Autodesk Fusion 360 part; units mm, degrees
sketch "Sketch1" plane through (0, 0, 0) normal (0, 0, 1) x (1, 0, 0)
  line L0 (0, 0) -> (35, 0)
  line L1 (35, 0) -> (35, 35)
  line L2 (35, 35) -> (0, 35)
  line L3 (0, 35) -> (0, 0)
  dimension "d1" = 35
  dimension "d2" = 35
extrude "Extrude1" add sketch "Sketch1" along normal blind 3
sketch "Sketch2" plane through (0, 0, 3) normal (0, 0, 1) x (-1, 0, 0)
  line L0 (0, -35) -> (0, 0)
  line L1 (0, 0) -> (-35, 0)
  line L2 (-35, 0) -> (-35, -35)
  line L3 (-35, -35) -> (0, -35)
  line L4 (-10, -35) -> (-35, -35)
  line L5 (-35, -35) -> (-35, -17.5)
  line L6 (-35, -17.5) -> (-10, -17.5)
  line L7 (-10, -17.5) -> (-10, -35)
  dimension "d5" = 25
  dimension "d6" = 17.5
extrude "Extrude2" cut sketch "Sketch2" against normal blind 3 contours L2 L3 L4 L5 L6 L7
sketch "Sketch6" plane through (0, 0, 3) normal (0, 0, 1) x (-1, 0, 0)
  line L0 (-35, -17.5) -> (-10, -17.5)
  line L1 (-10, -17.5) -> (-10, -35)
  line L2 (-10, -35) -> (0, -35)
  line L3 (0, -35) -> (0, 0)
  line L4 (0, 0) -> (-35, 0)
  line L5 (-35, 0) -> (-35, -17.5)
  line L6 (-10, -17.5) -> (-14, -17.5)
  line L7 (-14, -17.5) -> (-14, 0)
  line L8 (-14, 0) -> (-10, 0)
  line L9 (-10, 0) -> (-10, -17.5)
  dimension "d23" = 4
  dimension "d24" = 17.5
extrude "Extrude6" add sketch "Sketch6" along normal blind 6 contours L0 L4 L6 L7 L8 L9
extrude "Extrude7" cut 1 faces at (35, 5.8333, 1) along direction (-1, 0, 0) blind 5
sketch "Sketch7" plane through (0, 0, 3) normal (0, 0, 1) x (-1, 0, 0)
  line L0 (-30, 0) -> (-30, -17.5)
  line L1 (-30, -17.5) -> (-14, -17.5)
  line L2 (-14, -17.5) -> (-14, 0)
  line L3 (-14, 0) -> (-30, 0)
  line L4 (-30, -17.5) -> (-26, -17.5)
  line L5 (-26, -17.5) -> (-26, 0)
  line L6 (-26, 0) -> (-30, 0)
  line L7 (-30, 0) -> (-30, -17.5)
  dimension "d29" = 4
  dimension "d30" = 17.5
extrude "Extrude8" add sketch "Sketch7" along normal blind 6 contours L0 L1 L3 L4 L5 L6 L7
extrude "Extrude9" add 1 faces at (28.6667, 17.5, 4) along direction (0, 1, 0) blind 3.5
sketch "Sketch8" plane through (14, 0, 0) normal (1, 0, 0) x (0, 1, 0)
  line L0 (0, 3) -> (21, 3)
  line L1 (21, 3) -> (21, 9)
  line L2 (21, 9) -> (0, 9)
  line L3 (0, 9) -> (0, 3)
  line L4 (0, 7) -> (21, 7)
  line L5 (21, 7) -> (21, 5)
  line L6 (21, 5) -> (0, 5)
  line L7 (0, 5) -> (0, 7)
  dimension "d35" = 2
  dimension "d36" = 2
extrude "Extrude10" cut sketch "Sketch8" against normal blind 2 contours L1 L3 L4 L5 L6 L7
sketch "Sketch9" plane through (26, 0, 0) normal (-1, 0, 0) x (0, -1, 0)
  line L0 (-21, 3) -> (0, 3)
  line L1 (0, 3) -> (0, 9)
  line L2 (0, 9) -> (-21, 9)
  line L3 (-21, 9) -> (-21, 3)
  line L4 (-21, 7) -> (0, 7)
  line L5 (0, 7) -> (0, 5)
  line L6 (0, 5) -> (-21, 5)
  line L7 (-21, 5) -> (-21, 7)
  dimension "d39" = 2
  dimension "d40" = 2
extrude "Extrude11" cut sketch "Sketch9" against normal blind 2 contours L1 L3 L4 L5 L6 L7
sketch "Sketch10" plane through (0, 0, 5) normal (0, 0, 1) x (-1, 0, 0)
  line L0 (-26, -21) -> (-26, 0)
  line L1 (-26, 0) -> (-28, 0)
  line L2 (-28, 0) -> (-28, -21)
  line L3 (-28, -21) -> (-26, -21)
  line L4 (-26, 0) -> (-28, 0)
  line L5 (-28, 0) -> (-28, -2)
  line L6 (-28, -2) -> (-26, -2)
  line L7 (-26, -2) -> (-26, 0)
  dimension "d43" = 2
  dimension "d44" = 2
extrude "Extrude12" add sketch "Sketch10" along normal blind 2 contours L0 L1 L2 L4 L5 L6 L7
sketch "Sketch11" plane through (0, 0, 5) normal (0, 0, 1) x (-1, 0, 0)
  line L0 (-14, 0) -> (-14, -21)
  line L1 (-14, -21) -> (-12, -21)
  line L2 (-12, -21) -> (-12, 0)
  line L3 (-12, 0) -> (-14, 0)
  line L4 (-14, 0) -> (-12, 0)
  line L5 (-12, 0) -> (-12, -2)
  line L6 (-12, -2) -> (-14, -2)
  line L7 (-14, -2) -> (-14, 0)
  dimension "d47" = 2
  dimension "d48" = 2
extrude "Extrude13" add sketch "Sketch11" along normal blind 2 contours L0 L2 L3 L4 L5 L6 L7
sketch "Sketch14" plane through (0, 21, 0) normal (0, 1, 0) x (-1, 0, 0)
  line L0 (-26, 5) -> (-28, 5)
  line L1 (-28, 5) -> (-28, 7)
  line L2 (-28, 7) -> (-26, 7)
  line L3 (-26, 7) -> (-26, 9)
  line L4 (-26, 9) -> (-30, 9)
  line L5 (-30, 9) -> (-30, 0)
  line L6 (-30, 0) -> (-10, 0)
  line L7 (-10, 0) -> (-10, 3)
  line L8 (-10, 3) -> (-10, 9)
  line L9 (-10, 9) -> (-14, 9)
  line L10 (-14, 9) -> (-14, 7)
  line L11 (-14, 7) -> (-12, 7)
  line L12 (-12, 7) -> (-12, 5)
  line L13 (-12, 5) -> (-14, 5)
  line L14 (-14, 5) -> (-14, 3)
  line L15 (-14, 3) -> (-26, 3)
  line L16 (-26, 3) -> (-26, 5)
  line L17 (-10, 3) -> (-30, 3)
  line L18 (-30, 3) -> (-30, 0)
  line L19 (-30, 0) -> (-10, 0)
  line L20 (-10, 0) -> (-10, 3)
  dimension "d61" = 20
extrude "Extrude17" add sketch "Sketch14" along normal blind 10 contours L5 L6 L7 L15 L17 L18 L19 L20
extrude "Extrude18" cut 1 faces at (0, 23.3333, 1) along direction (1, 0, 0) blind 10
sketch "Sketch15" plane through (10, 0, 0) normal (-1, 0, 0) x (0, -1, 0)
  line L0 (0, 0) -> (0, 9)
  line L1 (0, 9) -> (-21, 9)
  line L2 (-21, 9) -> (-21, 3)
  line L3 (-21, 3) -> (-31, 3)
  line L4 (-31, 3) -> (-31, 0)
  line L5 (-31, 0) -> (0, 0)
  line L6 (-21, 3) -> (-31, 3)
  line L7 (-31, 3) -> (-31, 0)
  line L8 (-31, 0) -> (-21, 0)
  line L9 (-21, 0) -> (-21, 3)
extrude "Extrude19" add sketch "Sketch15" along normal blind 8 contours L3 L4 L5 L6 L7 L8 L9
sketch "Sketch16" plane through (30, 0, 0) normal (1, 0, 0) x (0, 1, 0)
  line L0 (21, 9) -> (0, 9)
  line L1 (0, 9) -> (0, 0)
  line L2 (0, 0) -> (31, 0)
  line L3 (31, 0) -> (31, 3)
  line L4 (31, 3) -> (21, 3)
  line L5 (21, 3) -> (21, 9)
  line L6 (21, 3) -> (31, 3)
  line L7 (31, 3) -> (31, 0)
  line L8 (31, 0) -> (21, 0)
  line L9 (21, 0) -> (21, 3)
  dimension "d68" = 10
extrude "Extrude20" add sketch "Sketch16" along normal blind 8 contours L2 L3 L4 L6 L7 L8 L9
sketch "Sketch17" plane through (0, 0, 0) normal (0, 0, -1) x (1, 0, 0)
  line L0 (10, 0) -> (10, -21)
  line L1 (10, -21) -> (2, -21)
  line L2 (2, -21) -> (2, -31)
  line L3 (2, -31) -> (38, -31)
  line L4 (38, -31) -> (38, -21)
  line L5 (38, -21) -> (30, -21)
  line L6 (30, -21) -> (30, 0)
  line L7 (30, 0) -> (10, 0)
  circle A0 centre (20, -26) radius 1.5
  dimension "d71" = 3
  dimension "d72" = 5
  dimension "d73" = 10
extrude "Extrude21" cut sketch "Sketch17" against normal blind 3 contours A0
sketch "Sketch18" plane through (0, 0, 0) normal (0, 0, -1) x (1, 0, 0)
  circle A0 centre (20, -26) radius 1.5
  line L0 (10, 0) -> (10, -21)
  line L1 (10, -21) -> (2, -21)
  line L2 (2, -21) -> (2, -31)
  line L3 (2, -31) -> (38, -31)
  line L4 (38, -31) -> (38, -21)
  line L5 (38, -21) -> (30, -21)
  line L6 (30, -21) -> (30, 0)
  line L7 (30, 0) -> (10, 0)
  circle A1 centre (6, -26) radius 1
  dimension "d76" = 2
  dimension "d77" = 14
extrude "Extrude22" cut sketch "Sketch18" against normal blind 3 contours A1
sketch "Sketch19" plane through (0, 0, 0) normal (0, 0, -1) x (1, 0, 0)
  circle A0 centre (6, -26) radius 1
  circle A1 centre (20, -26) radius 1.5
  line L0 (10, 0) -> (10, -21)
  line L1 (10, -21) -> (2, -21)
  line L2 (2, -21) -> (2, -31)
  line L3 (2, -31) -> (38, -31)
  line L4 (38, -31) -> (38, -21)
  line L5 (38, -21) -> (30, -21)
  line L6 (30, -21) -> (30, 0)
  line L7 (30, 0) -> (10, 0)
  circle A2 centre (34, -26) radius 1
  dimension "d80" = 2
  dimension "d81" = 14
  dimension "d82" = 5
extrude "Extrude23" cut sketch "Sketch19" against normal blind 3 contours A2
fillet "Fillet1" radius 5 1 edges at (38, 21, 1.5)
fillet "Fillet2" radius 5 1 edges at (38, 31, 1.5)
fillet "Fillet3" radius 5 1 edges at (2, 31, 1.5)
fillet "Fillet4" radius 5 1 edges at (2, 21, 1.5)
sketch "Sketch20" plane through (0, 0, 3) normal (0, 0, 1) x (-1, 0, 0)
  arc A0 (-7, -31) -> (-7, -21) centre (-7, -26) ccw
  line L0 (-7, -21) -> (-10, -21)
  line L1 (-10, -21) -> (-14, -21)
  line L2 (-14, -21) -> (-14, 0)
  line L3 (-14, 0) -> (-26, 0)
  line L4 (-26, 0) -> (-26, -21)
  line L5 (-26, -21) -> (-30, -21)
  line L6 (-30, -21) -> (-33, -21)
  arc A1 (-33, -21) -> (-33, -31) centre (-33, -26) ccw
  line L7 (-33, -31) -> (-7, -31)
  circle A2 centre (-34, -26) radius 1
  circle A3 centre (-6, -26) radius 1
  circle A4 centre (-20, -26) radius 1.5
  line L8 (-14, 0) -> (-26, 0)
  line L9 (-26, 0) -> (-26, -2)
  line L10 (-26, -2) -> (-14, -2)
  line L11 (-14, -2) -> (-14, 0)
  dimension "d93" = 2
extrude "Extrude24" add sketch "Sketch20" along normal blind 6 contours L2 L3 L4 L8 L9 L10 L11
extrude "Extrude25" add 1 faces at (28.6667, 7.6667, 9) along direction (0, 0, 1) blind 3
extrude "Extrude26" add 1 faces at (23.3333, 0, 8) along direction (0, -1, 0) blind 1
sketch "Sketch22" plane through (0, -1, 0) normal (0, -1, 0) x (1, 0, 0)
  line L0 (10, 12) -> (10, 0)
  line L1 (10, 0) -> (30, 0)
  line L2 (30, 0) -> (30, 12)
  line L3 (30, 12) -> (10, 12)
  circle A0 centre (20, 7) radius 4
  dimension "d104" = 8
  dimension "d105" = 5
  dimension "d106" = 10
extrude "Extrude27" cut sketch "Sketch22" against normal blind 2 contours A0
sketch "Sketch23" plane through (0, 1, 0) normal (0, -1, 0) x (1, 0, 0)
  circle A0 centre (20, 7) radius 4
  circle A1 centre (20, 7) radius 3
  dimension "d109" = 6
extrude "Extrude28" cut sketch "Sketch23" against normal blind 1 contours A1
sketch "Sketch24" plane through (0, 0, 12) normal (0, 0, 1) x (-1, 0, 0)
  line L0 (-30, 1) -> (-30, -21)
  line L1 (-30, -21) -> (-26, -21)
  line L2 (-26, -21) -> (-26, -2)
  line L3 (-26, -2) -> (-14, -2)
  line L4 (-14, -2) -> (-14, -21)
  line L5 (-14, -21) -> (-10, -21)
  line L6 (-10, -21) -> (-10, 1)
  line L7 (-10, 1) -> (-30, 1)
  line L8 (-26, -21) -> (-30, -21)
  line L9 (-30, -21) -> (-30, -2)
  line L10 (-30, -2) -> (-26, -2)
  line L11 (-26, -2) -> (-26, -21)
extrude "Extrude29" cut sketch "Sketch24" against normal blind 3 contours L0 L1 L2 L8 L9 L10 L11
sketch "Sketch25" plane through (0, 0, 12) normal (0, 0, 1) x (-1, 0, 0)
  line L0 (-30, -2) -> (-14, -2)
  line L1 (-14, -2) -> (-14, -21)
  line L2 (-14, -21) -> (-10, -21)
  line L3 (-10, -21) -> (-10, 1)
  line L4 (-10, 1) -> (-30, 1)
  line L5 (-30, 1) -> (-30, -2)
  line L6 (-10, -21) -> (-14, -21)
  line L7 (-14, -21) -> (-14, -2)
  line L8 (-14, -2) -> (-10, -2)
  line L9 (-10, -2) -> (-10, -21)
  dimension "d114" = 4
extrude "Extrude30" cut sketch "Sketch25" against normal blind 3 contours L1 L2 L3 L6 L7 L8 L9
fillet "Fillet5" radius 3 1 edges at (30, -1, 6)
fillet "Fillet6" radius 3 1 edges at (10, -1, 6)
Build history of the part. All positions in model axes, mm. A direction names the side the tool comes from. Give positions to 0.01 mm unless a question says otherwise; leave off trailing zeros. Order: outer loops, then holes, each group sorted by start corner. A loop starts at its lowest first (then second) coordinate and runs counter-clockwise, first axis right, second up. Notation, with made-up numbers: M -11.5,-29.5 L -4.5,-29.5 A31 cw -4.5,-2.5 Z; hole C -19,-1.75 d4. An arc over 180 degrees is marked long. Use one line per item in the form item = value.
Q1. Wall check: probe 1 along Z at (x, y) = (20, 0.05); probe 2 along X at (y, z) = (26, 1.15); probe 3 along Y at (x, z) = (20, 2.1). Give the ranges that are in metal, low to high.
Conclusion:
probe_1 = 0 to 3, 11 to 12
probe_2 = 2 to 5, 7 to 18.5, 21.5 to 33, 35 to 38
probe_3 = -1 to 24.5, 27.5 to 31
Q2. Slice it at B-B, the plane z = 1.75. State how many separate pieces and enclosed holes the cut face has, and give its area (3 significant figures).
Conclusion:
separate_pieces = 1
enclosed_holes = 3
area = 761 mm2
Q3. Slice it at A-A, the plane x = 20. Write the cut outline in (y, z), and give its area (3 significant figures).
Conclusion:
outline = M -1,0 L 24.5,0 L 24.5,3 L 2,3 L 2,4 L 1,4 L 1,3 L -1,3 Z; M -1,11 L 1,11 L 1,10 L 2,10 L 2,12 L -1,12 Z; M 27.5,0 L 31,0 L 31,3 L 27.5,3 Z
area = 92.0 mm2
Q4. Which spindle directions (+Z, -Z, +X, -X, +Y, -Y) get a long thin tool onto all of the face, cutting with end or side? Do faces 1 (the flat face through (12, 11, 9)), 2 (the cylindrical face through (16.8, 0, 4.6)), 3 (the flat face through (28, 12, 6)). Say none if no direction does.
Conclusion:
face_1 = +Z, +X, -X, +Y
face_2 = -Y
face_3 = +Y
Q5. Pull direction Y, two halves, no side cores. Call faces 4 (the cylindrical face through (36, 22, 2)), 5 (the cylindrical face through (34, 27, 1)), 6 (the flat face through (27, 12, 7)): released by +Y, released by -Y, zero draft, split by the parting line, or undercut.
Conclusion:
face_4 = released by -Y
face_5 = undercut
face_6 = zero draft
Q6. Pin check, flat tips, straight feed: P1, Ø2.5, axis at y = 12.5, z = 2.5, coming from the +X side; P2, Ø1.5, axis at x = 31.5, y = 12.5, coming from the +Z side; P3, Ø2.5, axis at x = 34, y = 26, coming from the +Z side; P4, Ø2, axis at x = 27.5, y = 9, coming from the +Z side. Stop position of each tip, or through.
Conclusion:
P1 = 30
P2 = through
P3 = 3
P4 = 9
Q7. Slice it at C-C, the plane y = 12. Write the cut outline in (x, z), and give its area (3 significant figures).
Conclusion:
outline = M 10,0 L 30,0 L 30,9 L 26,9 L 26,7 L 28,7 L 28,5 L 26,5 L 26,3 L 14,3 L 14,5 L 12,5 L 12,7 L 14,7 L 14,9 L 10,9 Z
area = 100 mm2
Q8. Slice it at D-D, the plane x = 34. Write the cut outline in (y, z), and give its area (3 significant figures).
Conclusion:
outline = M 21.1,0 L 25,0 L 25,3 L 21.1,3 Z; M 27,0 L 30.9,0 L 30.9,3 L 27,3 Z
area = 23.4 mm2
